from build123d import *

# Parameters (mm, degrees)
BOX002_W     = 10
BOX002_H     = 10
BOX002_DEPTH = 10
BOX003_W     = 10
BOX003_H     = 10
BOX003_DEPTH = 10
BOX001_W     = 10
BOX001_H     = 10
BOX001_DEPTH = 10
BOX_W        = 10
BOX_H        = 10
BOX_DEPTH    = 10


with BuildPart() as obj1:
    # Box002 → Box002 (new body)
    with BuildSketch(Plane(origin=(0, -10, -10), x_dir=(1, 0, 0), z_dir=(0, 0, 1))):
        with Locations((5, 5)):
            Rectangle(BOX002_W, BOX002_H)
    extrude(amount=BOX002_DEPTH)


with BuildPart() as fusion001:
    # Box003 → Box003 (new body)
    with BuildSketch(Plane(origin=(10, 0, -10), x_dir=(1, 0, 0), z_dir=(0, 0, 1))):
        with Locations((5, 5)):
            Rectangle(BOX003_W, BOX003_H)
    extrude(amount=BOX003_DEPTH)

    # Fusion001: union obj1
    add(obj1.part)


with BuildPart() as obj2:
    # Box001 → Box001 (new body)
    with BuildSketch(Plane.XY.offset(-10)):
        with Locations((5, 5)):
            Rectangle(BOX001_W, BOX001_H)
    extrude(amount=BOX001_DEPTH)


with BuildPart() as fusion002:
    # Box → Box (new body)
    with BuildSketch(Plane.XY):
        with Locations((5, 5)):
            Rectangle(BOX_W, BOX_H)
    extrude(amount=BOX_DEPTH)

    # Fusion: union obj2
    add(obj2.part)

    # Fusion002: union Fusion001
    add(fusion001.part)


solid = fusion002.part
Could you check a few things on this model? Use its own coordinates, in mm. A direction names the side the tool comes from. Coordinates: 2 decimals unless noted, no trailing zeros. Write each loop counter-clockwise with the first axis right and the second up, starting at its lowest first coordinate (ties: lowest second). Pieces come first, ordered by that corner, then holes. Notation, with made-up numbers: M 12,36 L 31,36 A20 cw 31,62 Z; hole C 39,28.25 d3. An arc over 180 degrees is marked long. One line per question, with ' | ' between items.
1) For pin 1 Ø5 at (x, z) = (2.5, 4.5) entering from -Y; pin 2 Ø5 at (x, y) = (16.5, 5) entering from +Z; pin 3 Ø3 at (y, z) = (7.5, 4.5) entering from +X, each with a flat end and sliding along its axis, tell me the tip position at first contact or that it passes through.
Checks:
pin 1: y = 0 | pin 2: z = 0 | pin 3: x = 10
2) Imagine slicing it at C-C, the plane x = 4.5. Write out the boundary of the cut face in (y, z), and give its area (3 significant figures).
Checks:
outline: M -10,-10 L 10,-10 L 10,10 L 0,10 L 0,0 L -10,0 Z | area: 300 mm²
3) I need wall thicknesses on probe 1 along Z at (x, y) = (11.5, 3.25); probe 2 along X at (y, z) = (2.25, 6.5). Which ranges of each line are inside material? Lowest first, please. Write a range as [from, to].
Checks:
probe 1: [-10, 0] | probe 2: [0, 10]
4) Imagine slicing it at B-B, the plane y = -3.75. Write out the boundary of the cut face in (x, z), and give its area (3 significant figures).
Checks:
outline: M 0,-10 L 10,-10 L 10,0 L 0,0 Z | area: 100 mm²
5) Imagine slicing it at A-A, the plane z = -8. Write out the boundary of the cut face in (x, y).
Checks:
outline: M 0,-10 L 10,-10 L 10,0 L 20,0 L 20,10 L 0,10 Z
6) For faces 1 (the face through (5, -5, 0)), 2 (the face through (8, 10, -2)), 3 (the face through (10, 5, 5)), 4 (the face through (10, -5, -5)), 5 (the face through (20, 5, -5)), which set-ups out of +Z, -Z, +X, -X, +Y, -Y let a thin tool reach every point of the face, with its end or its side?
Checks:
face 1: +Z, +X, -X, -Y | face 2: +Z, -Z, +X, -X, +Y | face 3: +Z, +X, +Y, -Y | face 4: +Z, -Z, +X, -Y | face 5: +Z, -Z, +X, +Y, -Y
